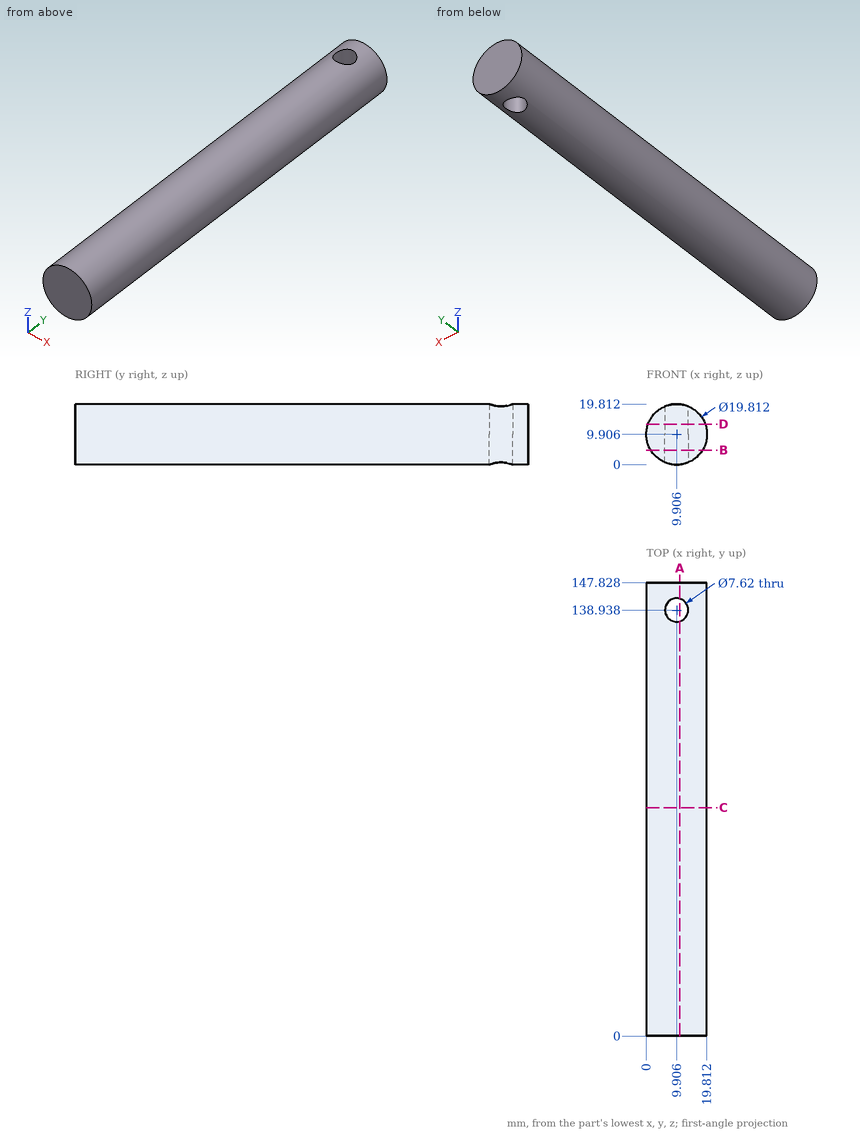
Could you check a few things on this drawing? It's one solid part, dimensions in mm from its lowest x, y, z. Round coordinates to 2 decimals unless told otherwise and drop trailing zeros. Write each loop counter-clockwise with the first axis right and the second up, starting at its lowest first coordinate (ties: lowest second). Pieces come first, ordered by that corner, then holes. Notation, with made-up numbers: (-12.75, -29.5) -> (22.25, -29.5) arc R8 cw to (22.25, -21.5) -> close; hole circle Ø2 at (68, 73.5). An arc over 180 degrees is marked (long way). Use one line per item in the form item = value. Start each with the question number.
Q1. Imagine slicing it at D-D (z = 13.25). Please give me the cut outline in (x, y), then the cut area to 3 significant figures.
Q2. Imagine slicing it at B-B (z = 4.75). Please give me the cut outline in (x, y).
Q3. Imagine slicing it at C-C (y = 74.5). Please give me the cut outline in (x, z).
Q4. Imagine slicing it at A-A (x = 11). Please give me the cut outline in (y, z).
Q5. I'm going to push flat-ended pins straight in: P1, Ø1.5, axis at x = 15, y = 56.5, coming from the -Z side; P2, Ø4.5, axis at x = 9.906, y = 138.938, coming from the -Z side; P3, Ø1.5, axis at y = 97, z = 6, coming from the -X side; P4, Ø10, axis at x = 16.5, y = 78.5, coming from the -Z side. Where does each tip first touch, or does it pass through?
Q6. If I drill on probe 1 along X at (y, z) = (24, 10.25); probe 2 along Y at (x, z) = (8.5, 4.5); probe 3 along Y at (x, z) = (13, 17.5), over which ranges is the centre line in solid material (lowest first)? Write a range as [from, to].
Worked out:
q1.outline = (0.58, 0) -> (19.23, 0) -> (19.23, 147.83) -> (0.58, 147.83) -> close; hole circle Ø7.62 at (9.91, 138.94)
q1.area = 2,710 mm^2
q2.outline = (1.45, 0) -> (18.36, 0) -> (18.36, 147.83) -> (1.45, 147.83) -> close; hole circle Ø7.62 at (9.91, 138.94)
q3.outline = circle Ø19.81 at (9.91, 9.91)
q4.outline = (0, 0.06) -> (135.29, 0.06) -> (135.29, 19.75) -> (0, 19.75) -> close; (142.59, 0.06) -> (147.83, 0.06) -> (147.83, 19.75) -> (142.59, 19.75) -> close
q5.P1 = 1
q5.P2 = through
q5.P3 = 0.52
q5.P4 = 0.13
q6.probe_1 = [0.01, 19.81]
q6.probe_2 = [0, 135.4], [142.48, 147.83]
q6.probe_3 = [0, 136.71], [141.16, 147.83]
